```python
from build123d import *

# Parameters (mm, degrees)
F0_W     = 200
F0_H     = 200
F1_DEPTH = 3


with BuildPart() as f1:
    # F0 (on Top) → F1 (new body)
    with BuildSketch(Plane.XY):
        with Locations((-0.150979, 12.599895)):
            Rectangle(F0_W, F0_H)
        Polygon((92.378985, -80.081508), (-89.743175, -80.081508), (1.317902, 9.357106), align=None, mode=Mode.SUBTRACT)
        Polygon((4.787778, 12.765158), (93.662091, 100.05597), (93.662091, -74.918876), align=None, mode=Mode.SUBTRACT)
        Polygon((-94.644882, -77.369233), (-94.644882, 103.610084), (-2.40064, 13.009393), align=None, mode=Mode.SUBTRACT)
        Polygon((1.081851, 16.421451), (-90.312292, 106.591567), (93.11328, 106.591567), align=None, mode=Mode.SUBTRACT)
    extrude(amount=F1_DEPTH)


solid = f1.part
```
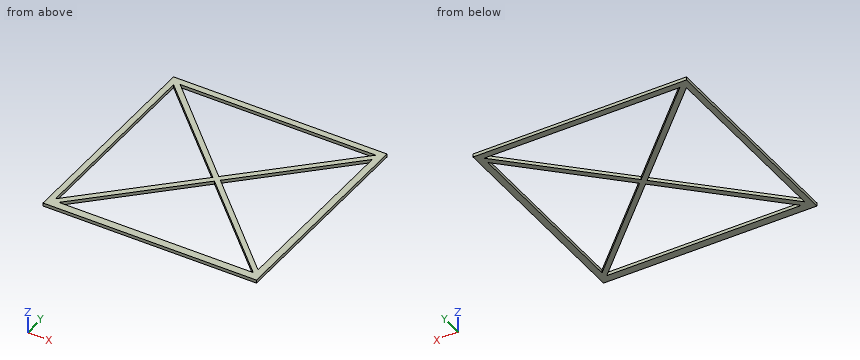
Model file for the job. Use its own axes, mm. Give positions to 0.01 mm unless a question says otherwise; leave off trailing zeros. Loops run counter-clockwise (first coordinate to the right, second up) from the corner with the lowest first, then second, coordinate; pieces in that order, holes last. Notation, with made-up numbers: (75.5, 45.25) - (116.5, 45.25) arc R32 cw to (116.5, 72.25) - close; hole circle Ø1 at (-31, 64). An arc over 180 degrees is marked (long way). One line per item, written item: value. Start each with the question number.
1. Slice it at C-C (y = -12). List the corners of the cut face in (x, z), plus the area to 3 significant figures.
2. Probe L1, parallel to X at y = 36, z = 1.35; L2, parallel to Y at x = 23, z = 2.8; L3, parallel to X at y = -31, z = 0.75. List the from-to ranges inside material, lowest first. Write a range as from..to.
3. Slice it at A-A (z = 2.4). List the corners of the cut face in (x, y), plus the area to 3 significant figures.
4. Slice it at B-B (x = -84). List the corners of the cut face in (y, z).
Solution:
1. outline: (-100.15, 0) - (-94.64, 0) - (-94.64, 3) - (-100.15, 3) - close; (-27.93, 0) - (-20.43, 0) - (-20.43, 3) - (-27.93, 3) - close; (23.06, 0) - (29.89, 0) - (29.89, 3) - (23.06, 3) - close; (93.66, 0) - (99.85, 0) - (99.85, 3) - (93.66, 3) - close
1. area: 78.1 mm^2
2. L1: x = -100.15..-94.64, -25.81..-18.76, 21.06..28.44, 93.66..99.85
2. L2: y = -87.4..-80.08, -11.94..-5.2, 30.65..37.9, 106.59..112.6
2. L3: x = -100.15..-94.64, -47.32..-39.77, 42.41..49.15, 93.66..99.85
3. outline: (-100.15, -87.4) - (99.85, -87.4) - (99.85, 112.6) - (-100.15, 112.6) - close; hole (-94.64, -77.37) - (-2.4, 13.01) - (-94.64, 103.61) - close; hole (-90.31, 106.59) - (1.08, 16.42) - (93.11, 106.59) - close; hole (-89.74, -80.08) - (92.38, -80.08) - (1.32, 9.36) - close; hole (4.79, 12.77) - (93.66, -74.92) - (93.66, 100.06) - close
3. area: 7,460 mm^2
4. outline: (-87.4, 0) - (-80.08, 0) - (-80.08, 3) - (-87.4, 3) - close; (-74.44, 0) - (-66.94, 0) - (-66.94, 3) - (-74.44, 3) - close; (93.15, 0) - (100.36, 0) - (100.36, 3) - (93.15, 3) - close; (106.59, 0) - (112.6, 0) - (112.6, 3) - (106.59, 3) - close
